from build123d import *

# Parameters (mm, degrees)
SKETCH_R      = 1.6
SKETCH_R_2    = 3
SKETCH_R_3    = 35
EXTRUDE_DEPTH = 3


with BuildPart() as part:
    # Sketch → Extrude (new body)
    with BuildSketch(Plane.XY):
        with BuildLine():
            Line((16.082868, 8), (230.156125, 8))
            ThreePointArc((230.156125, 8), (233.316389, 9.389315), (234.823147, 12.495299))
            Line((234.823147, 12.495299), (236.609086, 50))
            Line((236.609086, 50), (234.818635, 88.494692))
            ThreePointArc((234.818635, 88.494692), (233.286361, 91.630467), (230.076169, 93))
            Line((230.076169, 93), (16.126662, 93))
            ThreePointArc((16.126662, 93), (12.911047, 91.609366), (11.397447, 88.449769))
            Line((11.397447, 88.449769), (9.609086, 50))
            Line((9.609086, 50), (11.396507, 12.46415))
            ThreePointArc((11.396507, 12.46415), (12.919924, 9.371506), (16.082868, 8))
        make_face()
        with Locations((44.561357, 62.315305)):
            Circle(SKETCH_R, mode=Mode.SUBTRACT)
        with Locations((85.061357, 62.315305)):
            Circle(SKETCH_R, mode=Mode.SUBTRACT)
        with Locations((135.082868, 81)):
            Circle(SKETCH_R_2, mode=Mode.SUBTRACT)
        with Locations((197.082868, 81)):
            Circle(SKETCH_R_2, mode=Mode.SUBTRACT)
        with Locations((197.082868, 19)):
            Circle(SKETCH_R_2, mode=Mode.SUBTRACT)
        with Locations((135.082868, 19)):
            Circle(SKETCH_R_2, mode=Mode.SUBTRACT)
        with Locations((166.082868, 50)):
            Circle(SKETCH_R_3, mode=Mode.SUBTRACT)
        Polygon((78.811357, 66.315305), (72.811357, 72.315305), (56.811357, 72.315305), (50.811357, 66.315305), (50.811357, 52.315305), (78.811357, 52.315305), align=None, mode=Mode.SUBTRACT)
    extrude(amount=EXTRUDE_DEPTH)


solid = part.part
Input: part model. Units: mm. Frame: model coordinates. A direction names the side the tool comes from. Round coordinates to 2 decimals unless told otherwise and drop trailing zeros. Loops run counter-clockwise (first coordinate to the right, second up) from the corner with the lowest first, then second, coordinate; pieces in that order, holes last. Notation, with made-up numbers: (67, 53.5) -> (120, 53.5) arc R17 ccw to (120, 57.5) -> close; hole circle Ø8 at (68, 19.5). An arc over 180 degrees is marked (long way). Answer as a JSON object with one key per item and string values. Group by question number.
1) Draft query along X for faces 3 (the flat face through (53.853, 69.357, 1.479)), 4 (the cylindrical face through (233.281, 9.355, 1.479)), 5 (the cylindrical face through (12.88, 9.41, 1.48)), 6 (the flat face through (122, 51, 3)). Return one class per face: +X half, -X half, draft (parallel to the pull), parting line (faces both ways), or undercut.
2) Section query D-D on y = 57. Output: boundary loops of the cut face in (x, z).
3) Section query A-A on x = 167.5. Output: boundary loops of the cut face in (y, z).
4) Pin query (flat end, axial travel): pin 1 (0.9 mm diameter, centred on y = 57, z = 2, fed in from +X). Return the tip coordinate at first contact, or that it passes through.
5) Reachability of faces 1 (the flat face through (75.853, 69.273, 1.479)), 2 (the flat face through (122, 51, 0)) from +Z, -Z, +X, -X, +Y, -Y: full face, straight path, thin tool, end or side. Return the list, or none.
6) Ray query, L1, parallel to Y at x = 72.5, z = 0.75; L2, parallel to X at y = 54, z = 0.85; L3, parallel to X at y = 57, z = 1. Return the intervals inside material, ascending.
7) Section query C-C on z = 0.6. State how many separate pieces and enclosed holes the cut face has, plus the area to 3 significant figures.
8) Section query B-B on y = 81. Output: boundary loops of the cut face in (x, z).
Reply:
{
 "1": {"face 3": "undercut", "face 4": "+X half", "face 5": "-X half", "face 6": "draft"},
 "2": {"outline": "(9.93, 0) -> (50.81, 0) -> (50.81, 3) -> (9.93, 3) -> close; (78.81, 0) -> (131.79, 0) -> (131.79, 3) -> (78.81, 3) -> close; (200.38, 0) -> (236.28, 0) -> (236.28, 3) -> (200.38, 3) -> close"},
 "3": {"outline": "(8, 0) -> (15.03, 0) -> (15.03, 3) -> (8, 3) -> close; (84.97, 0) -> (93, 0) -> (93, 3) -> (84.97, 3) -> close"},
 "4": {"pin 1": "stops at x = 236.3"},
 "5": {"face 1": "+Z, -Z", "face 2": "-Z, +X, -X, +Y, -Y"},
 "6": {"L1": "y = 8 to 52.32, 72.32 to 93", "L2": "x = 9.8 to 50.81, 78.81 to 131.31, 200.85 to 236.42", "L3": "x = 9.93 to 50.81, 78.81 to 131.79, 200.38 to 236.28"},
 "7": {"separate pieces": "1", "enclosed holes": "8", "area": "14,600 mm2"},
 "8": {"outline": "(11.05, 0) -> (132.08, 0) -> (132.08, 3) -> (11.05, 3) -> close; (138.08, 0) -> (149.83, 0) -> (149.83, 3) -> (138.08, 3) -> close; (182.33, 0) -> (194.08, 0) -> (194.08, 3) -> (182.33, 3) -> close; (200.08, 0) -> (235.17, 0) -> (235.17, 3) -> (200.08, 3) -> close"}
}
